Geometry check sheet. Reference: the model listing, model coordinates, mm. Face numbers are marked on the shaded views. A direction names the side the tool comes from. Give positions to 0.01 mm unless a question says otherwise; leave off trailing zeros. Loops run counter-clockwise (first coordinate to the right, second up) from the corner with the lowest first, then second, coordinate; pieces in that order, holes last. Notation, with made-up numbers: (85, -13) -> (116, -13) arc R25 cw to (116, 3) -> close; hole circle Ø2 at (59, 5.5). An arc over 180 degrees is marked (long way). Write item = value, one per line.
```python
from build123d import *

# Parameters (mm, degrees)
SKETCH1_W           = 20
SKETCH1_H           = 58.42
SKETCH1_R           = 2.55
BOSS_EXTRUDE1_DEPTH = 7.9375
CUT_EXTRUDE1_DEPTH  = 63.256729004


with BuildPart() as part:
    # Sketch1 → Boss-Extrude1 (new body)
    with BuildSketch(Plane.XY):
        with Locations((10, 29.21)):
            Rectangle(SKETCH1_W, SKETCH1_H)
        with Locations((10, 52.78)):
            Circle(SKETCH1_R, mode=Mode.SUBTRACT)
        with Locations((10, 5.64)):
            Circle(SKETCH1_R, mode=Mode.SUBTRACT)
        with BuildLine():
            Line((13.25, 24.2975), (13.25, 34.1225))
            ThreePointArc((13.25, 34.1225), (14.372532015, 36.832532015), (11.6625, 35.71))
            Line((11.6625, 35.71), (8.3375, 35.71))
            ThreePointArc((8.3375, 35.71), (5.627467985, 36.832532015), (6.75, 34.1225))
            Line((6.75, 34.1225), (6.75, 24.2975))
            ThreePointArc((6.75, 24.2975), (5.627467985, 21.587467985), (8.3375, 22.71))
            Line((8.3375, 22.71), (11.6625, 22.71))
            ThreePointArc((11.6625, 22.71), (14.372532015, 21.587467985), (13.25, 24.2975))
        make_face(mode=Mode.SUBTRACT)
    extrude(amount=BOSS_EXTRUDE1_DEPTH)

    # Sketch2 → Cut-Extrude1 (cut, through all)
    with BuildSketch(Plane(origin=(20, 0, 0), x_dir=(0, 0, -1), z_dir=(1, 0, 0))):
        with BuildLine():
            Line((-7.9375, 33.26), (-7.9375, 25.16))
            ThreePointArc((-7.9375, 25.16), (-3.8875, 29.21), (-7.9375, 33.26))
        make_face()
    extrude(amount=-CUT_EXTRUDE1_DEPTH, mode=Mode.SUBTRACT)


solid = part.part
```
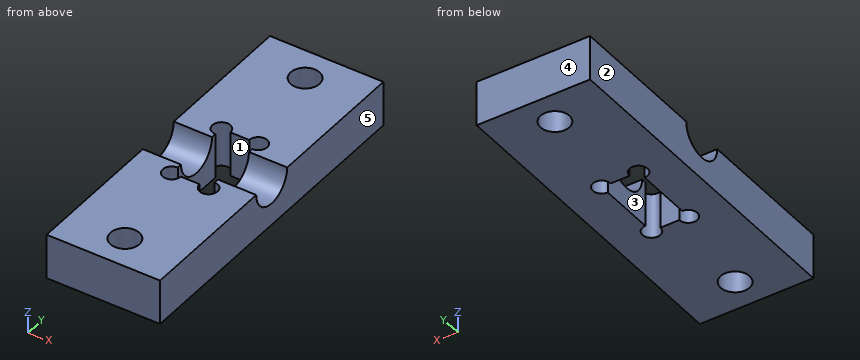
Item 1: Draft check along X on the marked faces 3, 4 and 5. Enter one of: +X half, -X half, draft (parallel to the pull), parting line (faces both ways), or undercut.
Answer:
face_3 = undercut
face_4 = draft
face_5 = +X half
Item 2: Section check C-C, the plane z = 2. Give the number of separate pieces and of enclosed holes in the cut face, plus the area to 3 significant figures.
Answer:
separate_pieces = 1
enclosed_holes = 3
area = 1,020 mm^2
Item 3: Thickness scan on L1, parallel to Y at x = 10, z = 5.25; L2, parallel to Y at x = 11, z = 6; L3, parallel to X at y = 30, z = 1.75. Record the ranges inside material, lowest first. Write a range as [from, to].
Answer:
L1 = [0, 3.09], [8.19, 22.71], [35.71, 50.23], [55.33, 58.42]
L2 = [0, 3.29], [7.99, 22.71], [35.71, 50.43], [55.13, 58.42]
L3 = [0, 6.75], [13.25, 20]
Item 4: Tool access check on the marked faces 1 and 2. Record the directions out of +Z, -Z, +X, -X, +Y, -Y that give a thin tool (end or side, any length) a straight path to the whole face; none if there is none.
Answer:
face_1 = +Z, -Z
face_2 = +Z, -Z, -X, +Y, -Y
Item 5: Section check A-A, the plane x = 10. Record the cut outline in (y, z).
Answer:
outline = (0, 0) -> (3.09, 0) -> (3.09, 7.94) -> (0, 7.94) -> close; (8.19, 0) -> (22.71, 0) -> (22.71, 7.94) -> (8.19, 7.94) -> close; (35.71, 0) -> (50.23, 0) -> (50.23, 7.94) -> (35.71, 7.94) -> close; (55.33, 0) -> (58.42, 0) -> (58.42, 7.94) -> (55.33, 7.94) -> close
Item 6: Section check B-B, the plane y = 29.21. Record the cut outline in (x, z).
Answer:
outline = (0, 0) -> (6.75, 0) -> (6.75, 3.89) -> (0, 3.89) -> close; (13.25, 0) -> (20, 0) -> (20, 3.89) -> (13.25, 3.89) -> close
Item 7: Section check D-D, the plane y = 5.64. Record the cut outline in (x, z).
Answer:
outline = (0, 0) -> (7.45, 0) -> (7.45, 7.94) -> (0, 7.94) -> close; (12.55, 0) -> (20, 0) -> (20, 7.94) -> (12.55, 7.94) -> close
Item 8: Gauge pin test, flat end, axial feed: pin 1 (2.5 mm diameter, centred on x = 13.25, y = 35.71, fed in from +Z). Record the tip position at first contact, or that the pin passes through.
Answer:
pin_1 = through
